Here's how the part is built. I have some questions about the finished solid (model axes, mm). A direction names the side the tool comes from. Give positions to 0.01 mm unless a question says otherwise; leave off trailing zeros. Order: outer loops, then holes, each group sorted by start corner. A loop starts at its lowest first (then second) coordinate and runs counter-clockwise, first axis right, second up.
from build123d import *
from OCP.BRepFilletAPI import BRepFilletAPI_MakeChamfer

# Parameters (mm, degrees)
BOSS_EXTRUDE1_DEPTH     = 12.7
CUT_EXTRUDE1_DEPTH      = 37.367265501
CUT_EXTRUDE1_DEPTH_BACK = 3.81
CUT_EXTRUDE2_DEPTH      = 38.86900643
SKETCH4_R               = 1.5875
CUT_EXTRUDE3_DEPTH      = 29.765990614
SKETCH5_R               = 3.175
CUT_EXTRUDE4_DEPTH      = 6.35
CHAMFER1_SIZE           = 1.016
CHAMFER2_SIZE           = 5.08
CHAMFER2_SIZE2          = 2.932939367


with BuildPart() as part:
    # Sketch1 → Boss-Extrude1 (new body)
    with BuildSketch(Plane.XY):
        with BuildLine():
            Line((-6.096, 4.572), (-6.096, -33.528))
            Line((-6.096, -33.528), (6.096, -33.528))
            Line((6.096, -33.528), (6.096, 4.572))
            ThreePointArc((6.096, 4.572), (0, 7.62), (-6.096, 4.572))
        make_face()
    extrude(amount=BOSS_EXTRUDE1_DEPTH)

    # Sketch2 → Cut-Extrude1 (cut, two sides: drawn at the far end of the back side and taken through both)
    with BuildSketch(Plane.XY.offset(12.7).offset(-CUT_EXTRUDE1_DEPTH_BACK)):
        with BuildLine():
            Line((3.291584227, -0.262063492), (2.025590294, -16.163269841))
            ThreePointArc((2.025590294, -16.163269841), (0, -18.034), (-2.025590294, -16.163269841))
            Line((-2.025590294, -16.163269841), (-3.291584227, -0.262063492))
            ThreePointArc((-3.291584227, -0.262063492), (0, 3.302), (3.291584227, -0.262063492))
        make_face()
    extrude(amount=CUT_EXTRUDE1_DEPTH + CUT_EXTRUDE1_DEPTH_BACK, mode=Mode.SUBTRACT)

    # Sketch3 → Cut-Extrude2 (cut, through all)
    with BuildSketch(Plane(origin=(6.096, 0, 0), x_dir=(0, 0, -1), z_dir=(1, 0, 0))):
        Polygon((-12.7, -33.528), (-12.7, -26.67), (0, -23.368), (0, -33.528), align=None)
    extrude(amount=-CUT_EXTRUDE2_DEPTH, mode=Mode.SUBTRACT)

    # Sketch4 → Cut-Extrude3 (cut, through all)
    with BuildSketch(Plane.XY.offset(8.89)):
        Circle(SKETCH4_R)
    extrude(amount=-CUT_EXTRUDE3_DEPTH, mode=Mode.SUBTRACT)

    # Sketch5 → Cut-Extrude4 (cut)
    with BuildSketch(Plane(origin=(0, 0, 0), x_dir=(-1, 0, 0), z_dir=(0, 0, -1))):
        Circle(SKETCH5_R)
    extrude(amount=-CUT_EXTRUDE4_DEPTH, mode=Mode.SUBTRACT)

    # Chamfer1
    chamfer1_edges = [part.edges().sort_by_distance(p)[0] for p in [
        (3.175, 0, 6.35),
    ]]
    chamfer(chamfer1_edges, length=CHAMFER1_SIZE)

    # Chamfer2: one chamfer whose edges measure the first distance from different faces: ONE call of the kernel's chamfer builder (chamfer() names one face for all edges)
    chamfer2_edges_1 = [part.edges().sort_by_distance(p)[0] for p in [
        (-6.096, -25.019, 6.35),
    ]]
    chamfer2_side_1 = [part.faces().sort_by_distance(p)[0] for p in [
        (-6.096, -10.238852647, 6.468097282),
    ]]
    chamfer2_edges_2 = [part.edges().sort_by_distance(p)[0] for p in [
        (6.096, -25.019, 6.35),
    ]]
    chamfer2_side_2 = [part.faces().sort_by_distance(p)[0] for p in [
        (6.096, -10.238852647, 6.468097282),
    ]]
    chamfer2 = BRepFilletAPI_MakeChamfer(part.part.solid().wrapped)
    for e in chamfer2_edges_1:
        chamfer2.Add(CHAMFER2_SIZE, CHAMFER2_SIZE2, e.wrapped, chamfer2_side_1[0].wrapped)  # the first distance lies on this face
    for e in chamfer2_edges_2:
        chamfer2.Add(CHAMFER2_SIZE, CHAMFER2_SIZE2, e.wrapped, chamfer2_side_2[0].wrapped)  # the first distance lies on this face
    add(Compound.cast(chamfer2.Shape()), mode=Mode.REPLACE)


solid = part.part
Q1. If we section it at B-B on z = 8.25: List the corners of the cut face in (x, y) for me (1 decimal), plus the area to 3 significant figures.
Filled sheet:
outline: (-6.1, -20.3) - (-3.2, -25.5) - (3.2, -25.5) - (6.1, -20.3) - (6.1, 4.6) arc R7.6 ccw to (-6.1, 4.6) - close; hole circle Ø3.2 at (0, 0)
area: 369 mm2
Q2. I need wall thicknesses on L1, parallel to X at y = 0, z = 10.95; L2, parallel to Z at x = -2.5, y = -8; L3, parallel to X at y = -5.5, z = 9.5. Which ranges of each line are inside material? Lowest first, please.
Filled sheet:
L1: x = -6.1 to -3.3, 3.3 to 6.1
L2: z = 0 to 8.89
L3: x = -6.1 to -2.87, 2.87 to 6.1
Q3. For faces 5 (the face through (0.044, -25.042, 6.439)), 6 (the face through (0, -7, 8.89)), 7 (the face through (0, 2, 6.35)), which set-ups out of +Z, -Z, +X, -X, +Y, -Y let a thin tool reach every point of the face, with its end or its side?
Filled sheet:
face 5: -Z, +X, -X, -Y
face 6: +Z
face 7: -Z
Q4. I'm going to push flat-ended pins straight in: P1, Ø1.5, axis at x = 0, y = -2, coming from the -Z side; P2, Ø3, axis at x = -1, z = 6.5, coming from the -Y side; P3, Ø2, axis at x = -1, y = -1, coming from the -Z side. Where does each tip first touch, or does it pass through?
Filled sheet:
P1: stops at z = 5.76
P2: stops at y = -25.45
P3: stops at z = 6.09
Q5. If we section it at C-C on y = -15.5: List the corners of the cut face in (x, z) for me, plus the area to 3 significant figures.
Filled sheet:
outline: (-6.1, 0) - (6.1, 0) - (6.1, 12.7) - (2.08, 12.7) - (2.08, 8.89) - (-2.08, 8.89) - (-2.08, 12.7) - (-6.1, 12.7) - close
area: 139 mm2
Q6. If we section it at D-D on z = 3: List the corners of the cut face in (x, y) for me (3 decimals).
Filled sheet:
outline: (-6.096, -18.899) - (-3.163, -24.148) - (3.163, -24.148) - (6.096, -18.899) - (6.096, 4.572) arc R7.62 ccw to (-6.096, 4.572) - close; hole circle Ø6.35 at (0, 0)
Q7. Thinking about a two-plate mould opening in X: for faces 1 (the face through (-2.65, -8.32, 10.77)), 2 (the face through (4.61, -22.45, 6.44)), 3 (the face through (0.1, 7.62, 6.26)), 4 (the face through (0, -8, 0)), which applies, released by +X, released by -X, zero draft, split by the parting line, or undercut?
Filled sheet:
face 1: undercut
face 2: released by +X
face 3: split by the parting line
face 4: zero draft
